Design review of the part built by this model. Coordinates are the model's own, in mm. A direction names the side the tool comes from. Give positions to 0.01 mm unless a question says otherwise; leave off trailing zeros.
```python
from build123d import *
from OCP.BRepFilletAPI import BRepFilletAPI_MakeChamfer

# Parameters (mm, degrees)
BOSS_EXTRUDE5_DEPTH = 50.8
FILLET9_R           = 5
CHAMFER1_SIZE       = 1
SKETCH8_R           = 1.35
BOSS_EXTRUDE6_DEPTH = 5
CUT_EXTRUDE3_DEPTH  = 20
CHAMFER2_SIZE       = 20
CHAMFER2_SIZE_2     = 0.69841539
SKETCH15_R          = 1.35
CUT_EXTRUDE4_DEPTH  = 5


with BuildPart() as part:
    # Sketch2 → Boss-Extrude5 (new body)
    with BuildSketch(Plane.XY):
        with BuildLine():
            Line((46.625, 27.5), (-46.625, 27.5))
            ThreePointArc((-46.625, 27.5), (-53.017219792, 25.190222762), (-56.456518829, 19.327905227))
            ThreePointArc((-56.456518829, 19.327905227), (-58.238005123, 0), (-56.456518829, -19.327905227))
            ThreePointArc((-56.456518829, -19.327905227), (-53.017219792, -25.190222762), (-46.625, -27.5))
            Line((-46.625, -27.5), (46.625, -27.5))
            ThreePointArc((46.625, -27.5), (53.017219792, -25.190222762), (56.456518829, -19.327905227))
            ThreePointArc((56.456518829, -19.327905227), (58.238005123, 0), (56.456518829, 19.327905227))
            ThreePointArc((56.456518829, 19.327905227), (53.017219792, 25.190222762), (46.625, 27.5))
        make_face()
    extrude(amount=BOSS_EXTRUDE5_DEPTH)

    # Fillet9
    fillet9_edges = [part.edges().sort_by_distance(p)[0] for p in [
        (53.017219792, -25.190222762, 50.8),
        (58.238005123, 0, 50.8),
        (53.017219792, 25.190222762, 50.8),
        (0, 27.5, 50.8),
        (-53.017219792, 25.190222762, 50.8),
        (-58.238005123, 0, 50.8),
        (-53.017219792, -25.190222762, 50.8),
        (0, -27.5, 50.8),
    ]]
    fillet(fillet9_edges, radius=FILLET9_R)

    # Chamfer1
    chamfer1_edges = [part.edges().sort_by_distance(p)[0] for p in [
        (58.238005123, 0, 0),
        (53.017219792, -25.190222762, 0),
        (0, -27.5, 0),
        (-53.017219792, -25.190222762, 0),
        (-58.238005123, 0, 0),
        (-53.017219792, 25.190222762, 0),
        (0, 27.5, 0),
        (53.017219792, 25.190222762, 0),
    ]]
    chamfer(chamfer1_edges, length=CHAMFER1_SIZE)

    # Sketch8 → Boss-Extrude6 (add)
    # profile 1 of 2: a face of its own
    with BuildSketch(Plane(origin=(18.825019181, 0, 0), x_dir=(0, 0, -1), z_dir=(1, 0, 0))):
        with BuildLine():
            Line((-13.405087735, -32.61), (-8.405087735, -27.5))
            Line((-8.405087735, -27.5), (-13.405087735, -27.5))
            Line((-13.405087735, -27.5), (-33.413673421, -27.5))
            Line((-33.413673421, -27.5), (-38.413673421, -27.5))
            Line((-38.413673421, -27.5), (-33.405087735, -32.61))
            Line((-33.405087735, -32.61), (-33.405087735, -42.61))
            ThreePointArc((-33.405087735, -42.61), (-23.405087735, -52.61), (-13.405087735, -42.61))
            Line((-13.405087735, -42.61), (-13.405087735, -32.61))
        make_face()
        with BuildLine():
            ThreePointArc((-33.105086536, -42.61), (-23.405087735, -32.910001198), (-13.705088933, -42.61))
            ThreePointArc((-13.705088933, -42.61), (-23.405087735, -52.309998802), (-33.105086536, -42.61))
        make_face(mode=Mode.SUBTRACT)
    # profile 2 of 2: a face of its own
    with BuildSketch(Plane(origin=(18.825019181, 0, 0), x_dir=(0, 0, -1), z_dir=(1, 0, 0))):
        with BuildLine():
            ThreePointArc((-33.105086536, -42.61), (-23.405087735, -52.309998802), (-13.705088933, -42.61))
            ThreePointArc((-13.705088933, -42.61), (-23.405087735, -32.910001198), (-33.105086536, -42.61))
        make_face()
        with Locations((-30.405089608, -42.61)):
            Circle(SKETCH8_R, mode=Mode.SUBTRACT)
        with Locations((-23.405087735, -49.610001873)):
            Circle(SKETCH8_R, mode=Mode.SUBTRACT)
        with Locations((-16.405085862, -42.61)):
            Circle(SKETCH8_R, mode=Mode.SUBTRACT)
        with Locations((-23.405087735, -35.609998127)):
            Circle(SKETCH8_R, mode=Mode.SUBTRACT)
        with BuildLine():
            ThreePointArc((-21.805087735, -42.61), (-23.405087735, -44.21), (-25.005087735, -42.61))
            ThreePointArc((-25.005087735, -42.61), (-23.405087735, -41.01), (-21.805087735, -42.61))
        make_face(mode=Mode.SUBTRACT)
    boss_extrude6 = extrude(amount=BOSS_EXTRUDE6_DEPTH)

    # Mirror1: Boss-Extrude6 across plane
    add(boss_extrude6.mirror(Plane(origin=(0, 0, 0), x_dir=(0, 0, 1), z_dir=(1, 0, 0))))

    # Sketch4 → Cut-Extrude3 (cut)
    with BuildSketch(Plane(origin=(0, 0, 0), x_dir=(-1, 0, 0), z_dir=(0, 0, -1))):
        with BuildLine():
            Line((-40.665, 14.165), (40.665, 14.165))
            ThreePointArc((40.665, 14.165), (44.200533906, 12.700533906), (45.665, 9.165))
            Line((45.665, 9.165), (45.665, -9.165))
            ThreePointArc((45.665, -9.165), (44.200533906, -12.700533906), (40.665, -14.165))
            Line((40.665, -14.165), (-40.665, -14.165))
            ThreePointArc((-40.665, -14.165), (-44.200533906, -12.700533906), (-45.665, -9.165))
            Line((-45.665, -9.165), (-45.665, 9.165))
            ThreePointArc((-45.665, 9.165), (-44.200533906, 12.700533906), (-40.665, 14.165))
        make_face()
    extrude(amount=-CUT_EXTRUDE3_DEPTH, mode=Mode.SUBTRACT)

    # Chamfer2
    chamfer2_edges_1 = [part.edges().sort_by_distance(p)[0] for p in [
        (-45.665, 0, 20),
    ]]
    chamfer2_side_1 = [part.faces().sort_by_distance(p)[0] for p in [
        (-45.665, 0, 19.986031692),
    ]]
    chamfer2_edges_2 = [part.edges().sort_by_distance(p)[0] for p in [
        (-44.200533906, 12.700533906, 20),
    ]]
    chamfer2_side_2 = [part.faces().sort_by_distance(p)[0] for p in [
        (-44.200533906, 12.700533906, 19.986031692),
    ]]
    chamfer2_edges_3 = [part.edges().sort_by_distance(p)[0] for p in [
        (-44.200533906, -12.700533906, 20),
    ]]
    chamfer2_side_3 = [part.faces().sort_by_distance(p)[0] for p in [
        (-44.200533906, -12.700533906, 19.986031692),
    ]]
    chamfer2_edges_4 = [part.edges().sort_by_distance(p)[0] for p in [
        (0, 14.165, 20),
    ]]
    chamfer2_side_4 = [part.faces().sort_by_distance(p)[0] for p in [
        (0, 14.165, 19.986031692),
    ]]
    chamfer2_edges_5 = [part.edges().sort_by_distance(p)[0] for p in [
        (0, -14.165, 20),
    ]]
    chamfer2_side_5 = [part.faces().sort_by_distance(p)[0] for p in [
        (0, -14.165, 19.986031692),
    ]]
    chamfer2_edges_6 = [part.edges().sort_by_distance(p)[0] for p in [
        (44.200533906, 12.700533906, 20),
    ]]
    chamfer2_side_6 = [part.faces().sort_by_distance(p)[0] for p in [
        (44.200533906, 12.700533906, 19.986031692),
    ]]
    chamfer2_edges_7 = [part.edges().sort_by_distance(p)[0] for p in [
        (44.200533906, -12.700533906, 20),
    ]]
    chamfer2_side_7 = [part.faces().sort_by_distance(p)[0] for p in [
        (44.200533906, -12.700533906, 19.986031692),
    ]]
    chamfer2_edges_8 = [part.edges().sort_by_distance(p)[0] for p in [
        (45.665, 0, 20),
    ]]
    chamfer2_side_8 = [part.faces().sort_by_distance(p)[0] for p in [
        (45.665, 0, 19.986031692),
    ]]
    chamfer2 = BRepFilletAPI_MakeChamfer(part.part.solid().wrapped)
    for e in chamfer2_edges_1:
        chamfer2.Add(CHAMFER2_SIZE - 0.0001, CHAMFER2_SIZE_2 - 0.0001, e.wrapped, chamfer2_side_1[0].wrapped)
    for e in chamfer2_edges_2:
        chamfer2.Add(CHAMFER2_SIZE - 0.0001, CHAMFER2_SIZE_2 - 0.0001, e.wrapped, chamfer2_side_2[0].wrapped)
    for e in chamfer2_edges_3:
        chamfer2.Add(CHAMFER2_SIZE - 0.0001, CHAMFER2_SIZE_2 - 0.0001, e.wrapped, chamfer2_side_3[0].wrapped)
    for e in chamfer2_edges_4:
        chamfer2.Add(CHAMFER2_SIZE - 0.0001, CHAMFER2_SIZE_2 - 0.0001, e.wrapped, chamfer2_side_4[0].wrapped)
    for e in chamfer2_edges_5:
        chamfer2.Add(CHAMFER2_SIZE - 0.0001, CHAMFER2_SIZE_2 - 0.0001, e.wrapped, chamfer2_side_5[0].wrapped)
    for e in chamfer2_edges_6:
        chamfer2.Add(CHAMFER2_SIZE - 0.0001, CHAMFER2_SIZE_2 - 0.0001, e.wrapped, chamfer2_side_6[0].wrapped)
    for e in chamfer2_edges_7:
        chamfer2.Add(CHAMFER2_SIZE - 0.0001, CHAMFER2_SIZE_2 - 0.0001, e.wrapped, chamfer2_side_7[0].wrapped)
    for e in chamfer2_edges_8:
        chamfer2.Add(CHAMFER2_SIZE - 0.0001, CHAMFER2_SIZE_2 - 0.0001, e.wrapped, chamfer2_side_8[0].wrapped)
    add(Compound.cast(chamfer2.Shape()), mode=Mode.REPLACE)  # a hair under: the kernel refuses the full size

    # Sketch15 → Cut-Extrude4 (cut)
    with BuildSketch(Plane(origin=(0, 0, 0), x_dir=(-1, 0, 0), z_dir=(0, 0, -1))):
        with Locations((-48.289265859, 18.560867196)):
            Circle(SKETCH15_R)
        with Locations((48.289265859, -18.560867196)):
            Circle(SKETCH15_R)
        with Locations((48.289265859, 18.560867196)):
            Circle(SKETCH15_R)
        with Locations((-48.289265859, -18.560867196)):
            Circle(SKETCH15_R)
    extrude(amount=-CUT_EXTRUDE4_DEPTH, mode=Mode.SUBTRACT)


solid = part.part
```
1. For line 1 along Y through (x, z) = (21, 41); line 2 along Z through (x, y) = (26.5, 12.5); line 3 along Y through (x, z) = (-49.5, 4.5), list the stretches that pass through material, from the lowest coordinate up.
Recorded:
line 1: y = -27.5 to 27.5
line 2: z = 20 to 50.8
line 3: y = -27.08 to -19.16, -17.96 to 17.96, 19.16 to 27.08
2. For pin 1 (4.5 mm diameter, centred on y = -42.61, z = 16.41, fed in from -X) (3 decimals); pin 2 (4 mm diameter, centred on x = 20.5, y = -36.5, fed in from +Z); pin 3 (4 mm diameter, centred on y = -4, z = 39, fed in from -X); pin 4 (4.5 mm diameter, centred on x = -48.29, y = -18.56, fed in from -Z), all flat-tipped, find the tip position at first contact; note any pin that passes through.
Recorded:
pin 1: stops at x = -23.825
pin 2: stops at z = 33.41
pin 3: stops at x = -58.22
pin 4: stops at z = 0
3. Machinability: for faces 1 (the face through (-18.825, -37, 24)), 2 (the face through (-43.9, 12.5, 10.1)), 3 (the face through (21.3, -36.4, 24.5)), which of the approach directions +Z, -Z, +X, -X, +Y, -Y give a long, thin tool a straight path to every point of the face, cutting with its end or side? Answer none if there is none.
Recorded:
face 1: +Z, -Z, -Y
face 2: -Z
face 3: +X, -X
4. Draft analysis for pull direction Y (two halves, no side actions). For faces 4 (the face through (21, -38, 13.405)), 5 (the face through (44, 12.4, 10.1)), 6 (the face through (53.09, 25.13, 23.09)), 7 (the face through (-21.29, -30.019, 35.944)), state which applies: pulls with the +Y half, pulls with the -Y half, needs draft (parallel to the pull), parting line crosses it, or undercut.
Recorded:
face 4: needs draft
face 5: undercut
face 6: pulls with the +Y half
face 7: pulls with the -Y half
